Can you work these out from the model? Positions are in its coordinate system, mm. A direction names the side the tool comes from. Give positions to 0.01 mm unless a question says otherwise; leave off trailing zeros. Write each loop counter-clockwise with the first axis right and the second up, starting at its lowest first coordinate (ties: lowest second). Pieces come first, ordered by that corner, then holes.
from build123d import *

# Parameters (mm, degrees)
SKETCH2_R              = 6.6929
BOSS_EXTRUDE1_DEPTH    = 15.113
SKETCH3_R              = 6.6929
BOSS_EXTRUDE2_DEPTH    = 4.62026
SKETCH4_R              = 7.9502
BOSS_EXTRUDE3_DEPTH    = 2.99974
M8X1_25_TAPPED_HOLE1_D = 6.8
CHAMFER2_SIZE          = 0.254


with BuildPart() as part:
    # Sketch2 → Boss-Extrude1 (new body)
    with BuildSketch(Plane(origin=(0, -87.315503791, 130.072474606), x_dir=(1, 0, 0), z_dir=(0, -0.557351153, 0.830276877))):
        with Locations((0, 484.511457201)):
            Circle(SKETCH2_R)
    extrude(amount=-BOSS_EXTRUDE1_DEPTH)

    # Sketch3 → Boss-Extrude2 (add)
    with BuildSketch(Plane(origin=(0, -87.315503791, 130.072474606), x_dir=(1, 0, 0), z_dir=(0, -0.557351153, 0.830276877))):
        with BuildLine():
            Line((-9.34974, 478.812023199), (-9.34974, 490.210891202))
            ThreePointArc((-9.34974, 490.210891202), (0, 495.461397201), (9.34974, 490.210891202))
            Line((9.34974, 490.210891202), (9.34974, 478.812023199))
            ThreePointArc((9.34974, 478.812023199), (0, 473.561517201), (-9.34974, 478.812023199))
        make_face()
        with Locations((0, 484.511457201)):
            Circle(SKETCH3_R, mode=Mode.SUBTRACT)
        with Locations((0, 484.511457201)):
            Circle(SKETCH3_R)
    extrude(amount=BOSS_EXTRUDE2_DEPTH)

    # Sketch4 → Boss-Extrude3 (add)
    with BuildSketch(Plane(origin=(0, -89.890611031, 133.908569648), x_dir=(1, 0, 0), z_dir=(0, -0.557351153, 0.830276877))):
        with Locations((0, 484.511457201)):
            Circle(SKETCH4_R)
    extrude(amount=BOSS_EXTRUDE3_DEPTH)

    # M8x1.25 Tapped Hole1 (through all)
    with Locations(Plane(origin=(0, -91.56251958, 136.399184405), x_dir=(1, 0, 0), z_dir=(0, -0.557351153, 0.830276877))):
        with Locations((0, 484.511457201)):
            Hole(M8X1_25_TAPPED_HOLE1_D / 2)

    # Chamfer2
    chamfer2_edges = [part.edges().sort_by_distance(p)[0] for p in [
        (-6.6929, 323.386403518, 387.567519724),
    ]]
    chamfer(chamfer2_edges, length=CHAMFER2_SIZE)


solid = part.part
(1) Will these pins go through, and if not, where does the flat tip stop? P1, Ø1.5, axis at x = -3, z = 395.5, coming from the +Y side; P2, Ø1.5, axis at y = 316.5, z = 393.5, coming from the -X side; P3, Ø1.5, axis at x = -2, y = 318.5, coming from the +Z side.
Returned:
P1: stops at y = 325.92
P2: stops at x = -6.48
P3: stops at z = 409.82
(2) If I drill on L1, parallel to Y at x = 1.75, z = 394.5; L2, parallel to X at y = 319.75, z = 394.75; L3, parallel to Z at x = 0.25, y = 304.75, over which ranges is the centre line in solid material (lowest first)?
Returned:
L1: y = 305.71 to 306.6, 310.95 to 315.22, 322.24 to 326.51
L2: x = -6.62 to -3.25, 3.25 to 6.62
L3: z = 395.69 to 398.82, 401.07 to 402.44
(3) Imagine slicing it at B-B, the plane z = 395.5. Give the number of separate pieces and of enclosed holes in the cut face, plus the area to 3 significant figures.
Returned:
separate pieces: 2
enclosed holes: 1
area: 157 mm2
(4) For faces 4 (the face through (0.157, 304.603, 395.904)), 5 (the face through (6.36, 316.56, 406.75)), which set-ups out of +Z, -Z, +X, -X, +Y, -Y let a thin tool reach every point of the face, with its end or its side?
Returned:
face 4: -Z, -Y
face 5: none
(5) Imagine slicing it at A-A, the plane x = 0. Write out the boundary of the cut face in (y, z), plus the area to 3 significant figures.
Returned:
outline: (303.3, 397.85) - (305.87, 394.01) - (309.41, 396.39) - (317.69, 384.05) - (318.04, 383.98) - (320.56, 385.67) - (307.89, 404.55) - (304.12, 402.01) - (305.79, 399.52) - close; (313.54, 408.34) - (326.21, 389.46) - (328.73, 391.16) - (328.8, 391.51) - (320.52, 403.85) - (324.05, 406.22) - (321.48, 410.05) - (318.99, 408.38) - (317.32, 410.87) - close
area: 197 mm2
(6) If we mould it in two halves opening along X, with no side actions, what happens to faces 1 (the face through (9.35, 314, 402)), 2 (the face through (0.737, 314.384, 395.023)), 3 (the face through (1.66, 307.87, 404.53))? For each: +X half, -X half, draft (parallel to the pull), parting line (faces both ways), or undercut.
Returned:
face 1: +X half
face 2: undercut
face 3: draft
